```python
from build123d import *

# Parameters (mm, degrees)
F0_W     = 263.190776
F0_H     = 95.95184
F1_DEPTH = 6.604
F2_W     = 49.028684
F2_H     = 95.95184
F3_DEPTH = 8.636
F4_R     = 4.891878
F5_DEPTH = 50.8


with BuildPart() as f1:
    # F0 (on Front) → F1 (new body)
    with BuildSketch(Plane.XZ):
        Rectangle(F0_W, F0_H)
    extrude(amount=F1_DEPTH)

    # F2 (on face) → F3 (join)
    with BuildSketch(Plane(origin=(0, 0, 0), x_dir=(-1, 0, 0), z_dir=(0, 1, 0))):
        Rectangle(F2_W, F2_H)
    extrude(amount=F3_DEPTH)

    # F4 (on face) → F5 (join)
    with BuildSketch(Plane(origin=(0, 0, -47.97592), x_dir=(1, 0, 0), z_dir=(0, 0, -1))):
        Circle(F4_R)
    extrude(amount=F5_DEPTH)


solid = f1.part
```
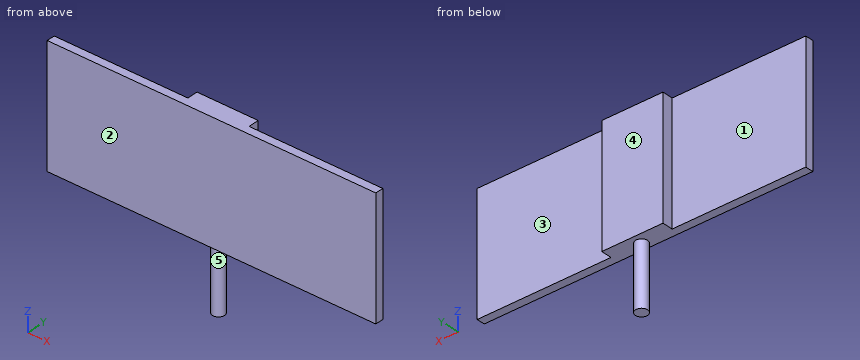
Work out the finished part from the listing and answer in its coordinate system (mm). Face numbers are marked on the shaded views. A direction names the side the tool comes from. Give positions to 0.01 mm unless a question says otherwise; leave off trailing zeros. Loops run counter-clockwise (first coordinate to the right, second up) from the corner with the lowest first, then second, coordinate; pieces in that order, holes last. Notation, with made-up numbers: (82.5, 14) -> (96.5, 14) arc R16 ccw to (96.5, 28) -> close; hole circle Ø11 at (60.5, 65.25). An arc over 180 degrees is marked (long way). Write item = value, one per line. Start each with the question number.
(1) Find section D-D on x = 10. Give the vertices of the cut face in (y, z), and give its area (3 significant figures).
(2) Given pin 1 Ø1.5 at (y, z) = (1, -6) entering from -X; pin 2 Ø7.5 at (x, y) = (27.5, -1) entering from -Z; pin 3 Ø4.5 at (y, z) = (5, 1.5) entering from +X, each flat-ended and moving along its own axis, determine where each tip first touches the part or whether it passes through.
(3) Find section C-C on x = 74. Give the vertices of the cut face in (y, z).
(4) Find section B-B on y = 2.5. Give the vertices of the cut face in (x, z), and give its area (3 significant figures).
(5) Find the intervals of material crossed by probe 1 along Z at (x, y) = (16, 3.25); probe 2 along Y at (x, z) = (-88, -8); probe 3 along X at (y, z) = (5.5, 9.5), in increasing order. Write a range as from..to.
(6) Which of the six approach directions +Z, -Z, +X, -X, +Y, -Y give full straight-line access (tool end or side, diameter ignored) to the marked faces 1, 2, 3, 4 and 5?
(7) Find section A-A on z = -14.5. Give the vertices of the cut face in (x, y), and give its area (3 significant figures).
From the geometry:
q1.outline = (-6.6, -47.98) -> (8.64, -47.98) -> (8.64, 47.98) -> (-6.6, 47.98) -> close
q1.area = 1,460 mm^2
q2.pin_1 = -24.51
q2.pin_2 = -47.98
q2.pin_3 = 24.51
q3.outline = (-6.6, -47.98) -> (0, -47.98) -> (0, 47.98) -> (-6.6, 47.98) -> close
q4.outline = (-24.51, -47.98) -> (-4.2, -47.98) -> (-4.2, -98.78) -> (4.2, -98.78) -> (4.2, -47.98) -> (24.51, -47.98) -> (24.51, 47.98) -> (-24.51, 47.98) -> close
q4.area = 5,130 mm^2
q5.probe_1 = -47.98..47.98
q5.probe_2 = -6.6..0
q5.probe_3 = -24.51..24.51
q6.face_1 = +Z, -Z, -X, +Y
q6.face_2 = +Z, -Z, +X, -X, -Y
q6.face_3 = +Z, -Z, +X, +Y
q6.face_4 = +Z, -Z, +X, -X, +Y
q6.face_5 = -Z
q7.outline = (-131.6, -6.6) -> (131.6, -6.6) -> (131.6, 0) -> (24.51, 0) -> (24.51, 8.64) -> (-24.51, 8.64) -> (-24.51, 0) -> (-131.6, 0) -> close
q7.area = 2,160 mm^2
